Build history of the part. All positions in model axes, mm. A direction names the side the tool comes from. Round coordinates to 2 decimals unless told otherwise and drop trailing zeros. Loops run counter-clockwise (first coordinate to the right, second up) from the corner with the lowest first, then second, coordinate; pieces in that order, holes last. Notation, with made-up numbers: (57, 37.5) - (87, 37.5) arc R7 cw to (87, 49.5) - close; hole circle Ø5 at (-36, 0.5). An arc over 180 degrees is marked (long way). Use one line per item in the form item = value. Start each with the question number.
Q1. Saw through at B-B (z = 4.5). Give the cut face in (x, y), then the cut area to 3 significant figures.
Q2. Saw through at A-A (z = -15). Give the cut face in (x, y), then the cut area to 3 significant figures.
Q3. Mould opens along Z. For faces 4 (the face through (-12.734, -4.01, -3.869)), 5 (the face through (-9, 0, -2)), 6 (the face through (0, 6, -20)) say: released by +Z, released by -Z, zero draft, split by the parting line, or undercut.
Q4. Pin check, flat tips, straight feed: pin 1 (5 mm diameter, centred on x = -9.5, y = 6, fed in from +Z); pin 2 (6 mm diameter, centred on x = -10.5, z = 0.5, fed in from +Y); pin 3 (0.8 mm diameter, centred on x = 0, y = -5.5, fed in from -Z). Stop position of each tip, or through.
Q5. Drill centre lines: line 1 (Y direction, x = 0, z = -21.3); line 2 (X direction, y = -0.5, z = -19); line 3 (Z direction, x = 5.25, y = 10). Where is each one in solid material? Low to high.
Q6. 3-axis set-ups, long thin cutter, end or side, ignore diameter. For faces 1 (the face through (-6.34, 12.2, -12.14)), 2 (the face through (8.25, 0.05, -0.99)), 3 (the face through (0.27, 4.78, -21.01)): which of +Z, -Z, +X, -X, +Y, -Y reach the whole face in a straight line?
```python
from build123d import *

# Parameters (mm, degrees)
SKETCH2_R           = 1.25
CUT_EXTRUDE1_DEPTH  = 2
SKETCH3_R           = 1.25
CUT_EXTRUDE2_DEPTH  = 2
SKETCH4_R           = 2.65
BOSS_EXTRUDE1_DEPTH = 1.2
SKETCH5_R           = 1.59
BOSS_EXTRUDE2_DEPTH = 9.2
CHAMFER1_SIZE       = 2


with BuildPart() as part:
    # Sketch1 → Revolve1 (revolve)
    with BuildSketch(Plane(origin=(0, 0, 0), x_dir=(1, 0, 0), z_dir=(0, 1, 0)), mode=Mode.PRIVATE) as revolve1_sk:
        Polygon((13.75, 0), (13.75, 3.666666667), (13.35, 3.666666667), (13.35, 4.066666667), (13.75, 4.066666667), (13.75, 22), (0, 22), (0, 0), align=None)
    revolve(revolve1_sk.sketch.rotate(Axis((0, 0, -22), (0, 0, 1)), 180), axis=Axis((0, 0, -22), (0, 0, 1)))

    # Sketch2 → Cut-Extrude1 (cut)
    with BuildSketch(Plane.XY):
        with Locations((9.5, 0)):
            Circle(SKETCH2_R)
        with Locations((0, 8)):
            Circle(SKETCH2_R)
        with Locations(Location((0, -8, 0), (0, 0, 180))):
            Circle(SKETCH2_R)
        with Locations(Location((-9.5, 0, 0), (0, 0, 180))):
            Circle(SKETCH2_R)
    extrude(amount=-CUT_EXTRUDE1_DEPTH, mode=Mode.SUBTRACT)

    # Sketch3 → Cut-Extrude2 (cut)
    with BuildSketch(Plane(origin=(0, 0, -22), x_dir=(-1, 0, 0), z_dir=(0, 0, -1))):
        with Locations((6, 0)):
            Circle(SKETCH3_R)
        with Locations((0, -6)):
            Circle(SKETCH3_R)
        with Locations((-6, 0)):
            Circle(SKETCH3_R)
        with Locations((0, 6)):
            Circle(SKETCH3_R)
    extrude(amount=-CUT_EXTRUDE2_DEPTH, mode=Mode.SUBTRACT)

    # Sketch4 → Boss-Extrude1 (add)
    with BuildSketch(Plane.XY):
        with Locations(Location((0, 0, 0), (0, 0, 180))):
            Circle(SKETCH4_R)
    extrude(amount=BOSS_EXTRUDE1_DEPTH)

    # Sketch5 → Boss-Extrude2 (add)
    with BuildSketch(Plane.XY.offset(1.2)):
        Circle(SKETCH5_R)
    extrude(amount=BOSS_EXTRUDE2_DEPTH)

    # Chamfer1
    chamfer1_edges = [part.edges().sort_by_distance(p)[0] for p in [
        (13.75, 0, -22),
    ]]
    chamfer(chamfer1_edges, length=CHAMFER1_SIZE)


solid = part.part
```
Report:
q1.outline = circle Ø3.18 at (0, 0)
q1.area = 7.94 mm²
q2.outline = circle Ø27.5 at (0, 0)
q2.area = 594 mm²
q3.face_4 = undercut
q3.face_5 = released by +Z
q3.face_6 = released by -Z
q4.pin_1 = 0
q4.pin_2 = 11.5
q4.pin_3 = -20
q5.line_1 = -12.45 to -7.25, -4.75 to 4.75, 7.25 to 12.45
q5.line_2 = -13.74 to 13.74
q5.line_3 = -22 to 0
q6.face_1 = +Z, -Z
q6.face_2 = +Z
q6.face_3 = -Z
